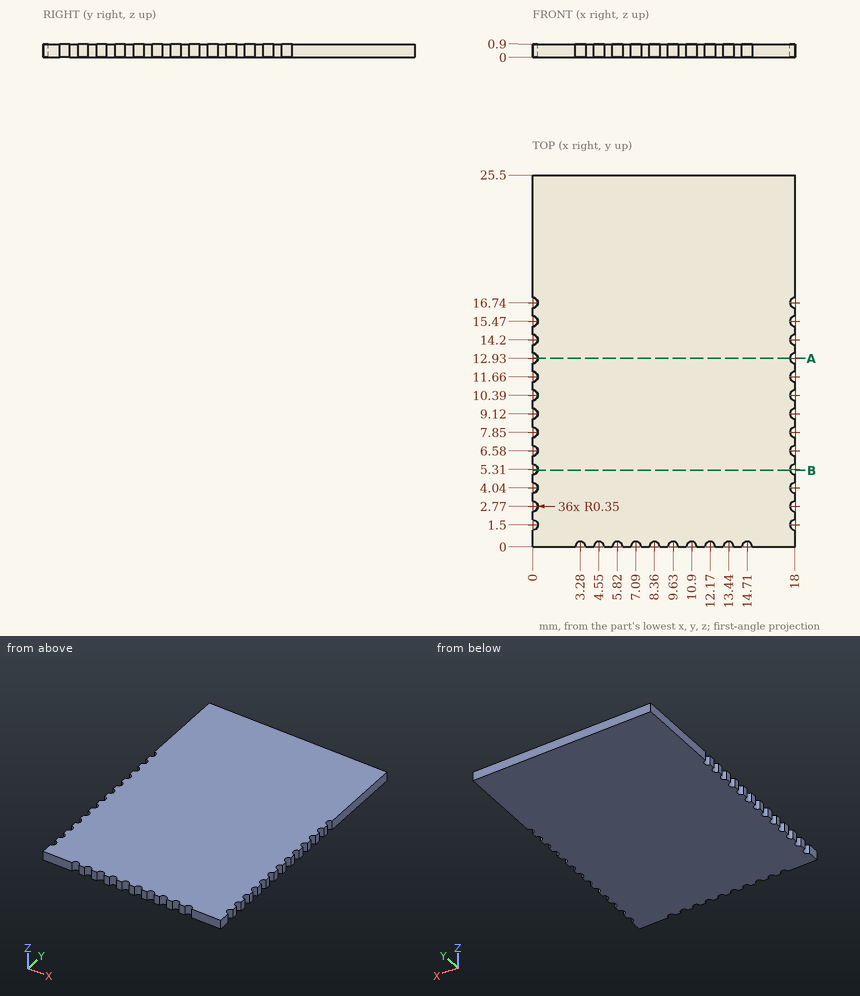
Answer from the drawing. Dimensions are ordinates in mm from the lowest x, y and z of the part. Round coordinates to 2 decimals unless told otherwise and drop trailing zeros. Write each loop counter-clockwise with the first axis right and the second up, starting at its lowest first coordinate (ties: lowest second). Pieces come first, ordered by that corner, then holes. Notation, with made-up numbers: (50.25, -13) -> (69.25, -13) arc R26 cw to (69.25, 13) -> close; hole circle Ø1 at (16.25, 65). An arc over 180 degrees is marked (long way). Answer in a Markdown table with one row per item. Add a question column.
1) Find section A-A, the plane y = 12.93. Determine the outline of the cut face in (x, z).
2) Consider line 1 (X direction, y = 13, z = 0.55); line 2 (Y direction, x = 4.5, z = 0.65); line 3 (Y direction, x = 3, z = 0.4). Determine where each line is inside the solid, lowest interval first.
3) Find section B-B, the plane y = 5.25. Determine the outline of the cut face in (x, z), and give its area (3 significant figures).
Findings below:
| question | item | result |
|---|---|---|
| 1 | outline | (0.35, 0) -> (17.65, 0) -> (17.65, 0.9) -> (0.35, 0.9) -> close |
| 2 | line 1 | 0.34 to 17.66 |
| 2 | line 2 | 0.35 to 25.5 |
| 2 | line 3 | 0.21 to 25.5 |
| 3 | outline | (0.34, 0) -> (17.66, 0) -> (17.66, 0.9) -> (0.34, 0.9) -> close |
| 3 | area | 15.6 mm² |
